CAD build for the part. Positions are in the model's coordinates, mm. A direction names the side the tool comes from. Give positions to 0.01 mm unless a question says otherwise; leave off trailing zeros. Write each loop counter-clockwise with the first axis right and the second up, starting at its lowest first coordinate (ties: lowest second). Pieces come first, ordered by that corner, then holes. Notation, with made-up numbers: (82.25, 13.5) - (114.25, 13.5) arc R6 cw to (114.25, 21.5) - close; hole circle Ø8 at (44.5, 16). An arc over 180 degrees is marked (long way). Write item = value, one per line. Start each with the question number.
```python
from build123d import *

# Parameters (mm, degrees)
BLOCK_DEPTH                    = 80
SHELL1_T                       = -3
SKETCH2_R                      = 5
CORNER_COLUMNS_DEPTH           = 80
SKETCH3_R                      = 2
FRONT_PANEL_INSERT_HOLES_DEPTH = 7
SKETCH4_R                      = 4.5
PLATE_BOSSES_DEPTH             = 6
SKETCH5_R                      = 2
PLATE_INSERT_HOLES_DEPTH       = 7
SKETCH6_R                      = 8.15
CABLE_GLAND_HOLES_DEPTH        = 4
SKETCH7_W                      = 12
SKETCH7_H                      = 6
CABLE_TIE_BARS_DEPTH           = 12
SKETCH8_W                      = 4
SKETCH8_H                      = 2.5
CABLE_TIE_SLOTS_DEPTH          = 6.02
SKETCH9_W                      = 14
SKETCH9_H                      = 14
USB_ACCESS_DEPTH               = 4
VENTS_LEFT_DEPTH               = 4
VENTS_START                    = -4
VENTS_RIGHT_DEPTH              = 4
SKETCH12_R                     = 4.75
KEYHOLE_HEADS_DEPTH            = 4
KEYHOLE_SLOTS_DEPTH            = 4
SKETCH14_W                     = 24
SKETCH14_H                     = 16
WALL_EARS_DEPTH                = 5
SKETCH15_R                     = 2.15
WALL_EAR_SCREW_HOLES_DEPTH     = 218.706224073


with BuildPart() as part:
    # Sketch1 → Block (new body)
    with BuildSketch(Plane.XY):
        with BuildLine():
            Line((-72, 0), (72, 0))
            ThreePointArc((72, 0), (77.656854249, 2.343145751), (80, 8))
            Line((80, 8), (80, 162))
            ThreePointArc((80, 162), (77.656854249, 167.656854249), (72, 170))
            Line((72, 170), (-72, 170))
            ThreePointArc((-72, 170), (-77.656854249, 167.656854249), (-80, 162))
            Line((-80, 162), (-80, 8))
            ThreePointArc((-80, 8), (-77.656854249, 2.343145751), (-72, 0))
        make_face()
    extrude(amount=BLOCK_DEPTH)

    # Shell1
    shell1_openings = [part.faces().sort_by_distance(p)[0] for p in [
        (0, 85, 80),
    ]]
    offset(amount=SHELL1_T, openings=shell1_openings, kind=Kind.INTERSECTION)

    # Sketch2 → Corner columns (add)
    with BuildSketch(Plane.XY):
        with Locations((-73, 7)):
            Circle(SKETCH2_R)
        with Locations((73, 7)):
            Circle(SKETCH2_R)
        with Locations((-73, 163)):
            Circle(SKETCH2_R)
        with Locations((73, 163)):
            Circle(SKETCH2_R)
    extrude(amount=CORNER_COLUMNS_DEPTH)

    # Sketch3 → Front panel insert holes (cut)
    with BuildSketch(Plane.XY.offset(80)):
        with Locations((-73, 7)):
            Circle(SKETCH3_R)
        with Locations((73, 7)):
            Circle(SKETCH3_R)
        with Locations((-73, 163)):
            Circle(SKETCH3_R)
        with Locations((73, 163)):
            Circle(SKETCH3_R)
    extrude(amount=-FRONT_PANEL_INSERT_HOLES_DEPTH, mode=Mode.SUBTRACT)

    # Sketch4 → Plate bosses (add)
    with BuildSketch(Plane.XY.offset(3)):
        with Locations((-57, 40)):
            Circle(SKETCH4_R)
        with Locations((57, 40)):
            Circle(SKETCH4_R)
        with Locations((-57, 150)):
            Circle(SKETCH4_R)
        with Locations((57, 150)):
            Circle(SKETCH4_R)
    extrude(amount=PLATE_BOSSES_DEPTH)

    # Sketch5 → Plate insert holes (cut)
    with BuildSketch(Plane.XY.offset(9)):
        with Locations((-57, 40)):
            Circle(SKETCH5_R)
        with Locations((57, 40)):
            Circle(SKETCH5_R)
        with Locations((-57, 150)):
            Circle(SKETCH5_R)
        with Locations((57, 150)):
            Circle(SKETCH5_R)
    extrude(amount=-PLATE_INSERT_HOLES_DEPTH, mode=Mode.SUBTRACT)

    # Sketch6 → Cable gland holes (cut)
    with BuildSketch(Plane(origin=(0, 0, 0), x_dir=(1, 0, 0), z_dir=(0, 1, 0))):
        with Locations(Location((-50, -40, 0), (0, 0, 270))):
            Circle(SKETCH6_R)
        with Locations(Location((0, -40, 0), (0, 0, 270))):
            Circle(SKETCH6_R)
        with Locations(Location((45, -40, 0), (0, 0, 270))):
            Circle(SKETCH6_R)
    extrude(amount=CABLE_GLAND_HOLES_DEPTH, mode=Mode.SUBTRACT)

    # Sketch7 → Cable tie bars (add)
    with BuildSketch(Plane.XY.offset(3)):
        with Locations((-50, 28)):
            Rectangle(SKETCH7_W, SKETCH7_H)
        with Locations((0, 28)):
            Rectangle(SKETCH7_W, SKETCH7_H)
        with Locations((45, 28)):
            Rectangle(SKETCH7_W, SKETCH7_H)
    extrude(amount=CABLE_TIE_BARS_DEPTH)

    # Sketch8 → Cable tie slots (cut)
    with BuildSketch(Plane(origin=(0, 24.99, 0), x_dir=(1, 0, 0), z_dir=(0, 1, 0))):
        with Locations((-50, -10)):
            Rectangle(SKETCH8_W, SKETCH8_H)
        with Locations((0, -10)):
            Rectangle(SKETCH8_W, SKETCH8_H)
        with Locations((45, -10)):
            Rectangle(SKETCH8_W, SKETCH8_H)
    extrude(amount=CABLE_TIE_SLOTS_DEPTH, mode=Mode.SUBTRACT)

    # Sketch9 → USB access (cut)
    with BuildSketch(Plane(origin=(-80, 0, 0), x_dir=(0, 0, -1), z_dir=(1, 0, 0))):
        with Locations((-18, 62)):
            Rectangle(SKETCH9_W, SKETCH9_H)
    extrude(amount=USB_ACCESS_DEPTH, mode=Mode.SUBTRACT)

    # Sketch10 → Vents left (cut)
    with BuildSketch(Plane(origin=(-80, 0, 0), x_dir=(0, 0, -1), z_dir=(1, 0, 0))):
        with BuildLine():
            Line((-20, 128.5), (-60, 128.5))
            ThreePointArc((-60, 128.5), (-61.5, 130), (-60, 131.5))
            Line((-60, 131.5), (-20, 131.5))
            ThreePointArc((-20, 131.5), (-18.5, 130), (-20, 128.5))
        make_face()
        with BuildLine():
            Line((-20, 136.5), (-60, 136.5))
            ThreePointArc((-60, 136.5), (-61.5, 138), (-60, 139.5))
            Line((-60, 139.5), (-20, 139.5))
            ThreePointArc((-20, 139.5), (-18.5, 138), (-20, 136.5))
        make_face()
        with BuildLine():
            Line((-20, 144.5), (-60, 144.5))
            ThreePointArc((-60, 144.5), (-61.5, 146), (-60, 147.5))
            Line((-60, 147.5), (-20, 147.5))
            ThreePointArc((-20, 147.5), (-18.5, 146), (-20, 144.5))
        make_face()
    extrude(amount=VENTS_LEFT_DEPTH, mode=Mode.SUBTRACT)

    # Sketch11 → Vents right (cut)
    with BuildSketch(Plane(origin=(80, 0, 0), x_dir=(0, 0, -1), z_dir=(1, 0, 0)).offset(VENTS_START)):
        with BuildLine():
            Line((-20, 128.5), (-60, 128.5))
            ThreePointArc((-60, 128.5), (-61.5, 130), (-60, 131.5))
            Line((-60, 131.5), (-20, 131.5))
            ThreePointArc((-20, 131.5), (-18.5, 130), (-20, 128.5))
        make_face()
        with BuildLine():
            Line((-20, 136.5), (-60, 136.5))
            ThreePointArc((-60, 136.5), (-61.5, 138), (-60, 139.5))
            Line((-60, 139.5), (-20, 139.5))
            ThreePointArc((-20, 139.5), (-18.5, 138), (-20, 136.5))
        make_face()
        with BuildLine():
            Line((-20, 144.5), (-60, 144.5))
            ThreePointArc((-60, 144.5), (-61.5, 146), (-60, 147.5))
            Line((-60, 147.5), (-20, 147.5))
            ThreePointArc((-20, 147.5), (-18.5, 146), (-20, 144.5))
        make_face()
    extrude(amount=VENTS_RIGHT_DEPTH, mode=Mode.SUBTRACT)

    # Sketch12 → Keyhole heads (cut)
    with BuildSketch(Plane.XY):
        with Locations((-40, 130)):
            Circle(SKETCH12_R)
        with Locations((40, 130)):
            Circle(SKETCH12_R)
    extrude(amount=KEYHOLE_HEADS_DEPTH, mode=Mode.SUBTRACT)

    # Sketch13 → Keyhole slots (cut)
    with BuildSketch(Plane.XY):
        with BuildLine():
            Line((-42.15, 130), (-42.15, 141))
            ThreePointArc((-42.15, 141), (-40, 143.15), (-37.85, 141))
            Line((-37.85, 141), (-37.85, 130))
            ThreePointArc((-37.85, 130), (-40, 127.85), (-42.15, 130))
        make_face()
        with BuildLine():
            Line((37.85, 130), (37.85, 141))
            ThreePointArc((37.85, 141), (40, 143.15), (42.15, 141))
            Line((42.15, 141), (42.15, 130))
            ThreePointArc((42.15, 130), (40, 127.85), (37.85, 130))
        make_face()
    extrude(amount=KEYHOLE_SLOTS_DEPTH, mode=Mode.SUBTRACT)

    # Sketch14 → Wall ears (add)
    with BuildSketch(Plane.XY):
        with Locations((-50, -8)):
            Rectangle(SKETCH14_W, SKETCH14_H)
        with Locations((-50, 178)):
            Rectangle(SKETCH14_W, SKETCH14_H)
        with Locations((50, -8)):
            Rectangle(SKETCH14_W, SKETCH14_H)
        with Locations((50, 178)):
            Rectangle(SKETCH14_W, SKETCH14_H)
    extrude(amount=WALL_EARS_DEPTH)

    # Sketch15 → Wall ear screw holes (cut, through all)
    with BuildSketch(Plane.XY):
        with Locations(Location((-50, -8, 0), (0, 0, 180))):
            Circle(SKETCH15_R)
        with Locations(Location((-50, 178, 0), (0, 0, 180))):
            Circle(SKETCH15_R)
        with Locations(Location((50, -8, 0), (0, 0, 180))):
            Circle(SKETCH15_R)
        with Locations(Location((50, 178, 0), (0, 0, 180))):
            Circle(SKETCH15_R)
    extrude(amount=WALL_EAR_SCREW_HOLES_DEPTH, mode=Mode.SUBTRACT)


solid = part.part
```
1. Pin check, flat tips, straight feed: pin 1 Ø8 at (x, y) = (-55.5, -8) entering from +Z; pin 2 Ø18.5 at (x, z) = (45, 40) entering from -Y; pin 3 Ø4.5 at (x, y) = (-57.5, 149.5) entering from +Z. Stop position of each tip, or through.
2. Tool access for faces 4 (the cylindrical face through (53.08, 1.48, 38.94)), 5 (the cylindrical face through (49.01, 179.91, 2.46)), 6 (the flat face through (39, 28, 9)): list every direction of +Z, -Z, +X, -X, +Y, -Y with a clear straight run to the whole face (end or side of a thin tool).
3. Mould opens along Y. For faces 1 (the flat face through (-77, 86, 41)), 2 (the flat face through (50, 186, 2)), 3 (the flat face through (38, 178, 2)) say: +Y half, -Y half, draft (parallel to the pull), parting line (faces both ways), or undercut.
4. Wall check: line 1 along Y through (x, z) = (50, 1); line 2 along Y through (x, z) = (51.5, 68); line 3 along X through (y, z) = (140, 33). Give the ranges that are in metal, low to high.
5. Cut at B-B (y = 88). Give the cut face in (x, z).
6. Cut at A-A (x = 25). Give the cut face in (y, z).
Output:
q1.pin_1 = 5
q1.pin_2 = 0
q1.pin_3 = 9
q2.face_4 = -Y
q2.face_5 = +Z, -Z
q2.face_6 = +Z
q3.face_1 = undercut
q3.face_2 = +Y half
q3.face_3 = draft
q4.line_1 = -16 to -10.15, -5.85 to 175.85, 180.15 to 186
q4.line_2 = 0 to 3, 167 to 170
q4.line_3 = -80 to -77, 77 to 80
q5.outline = (-80, 0) - (80, 0) - (80, 80) - (77, 80) - (77, 3) - (-77, 3) - (-77, 80) - (-80, 80) - close
q6.outline = (0, 0) - (170, 0) - (170, 80) - (167, 80) - (167, 3) - (3, 3) - (3, 80) - (0, 80) - close
